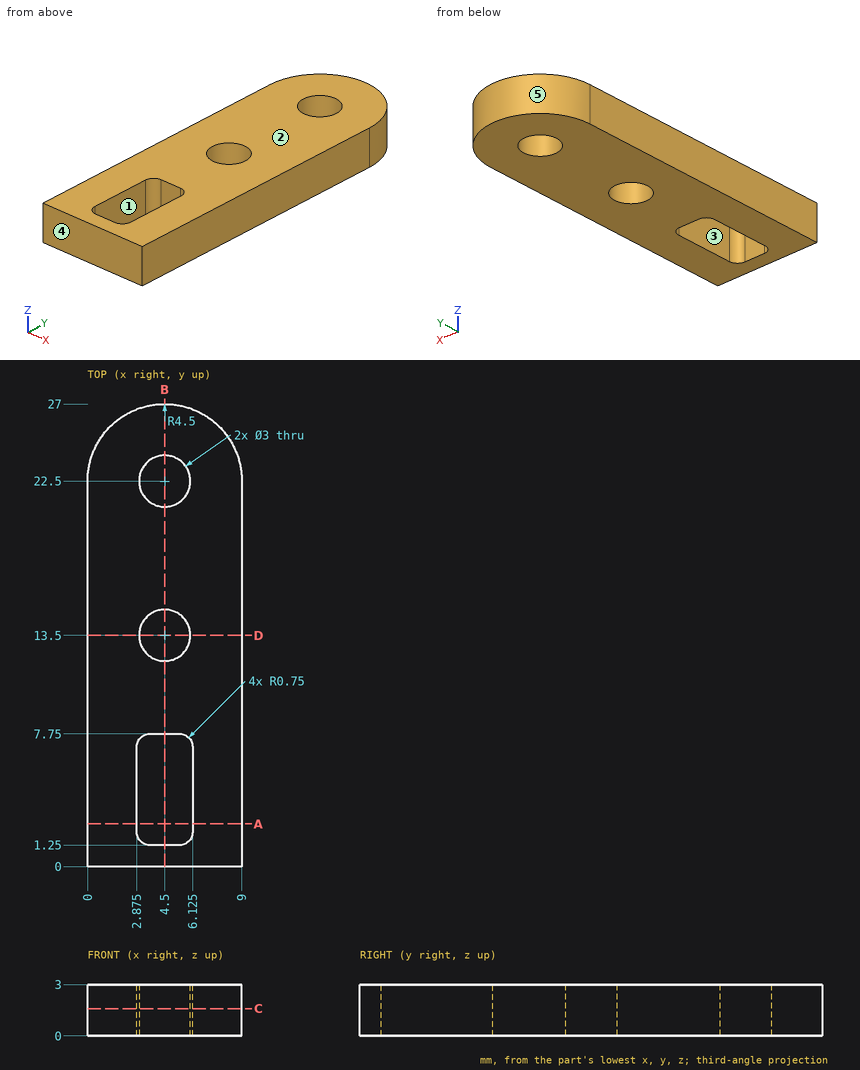
Here's the drawing with two shaded views (mm, measured from the low corner). I have some questions. A direction names the side the tool comes from. Coordinates: 2 decimals unless noted, no trailing zeros. Write each loop counter-clockwise with the first axis right and the second up, starting at its lowest first coordinate (ties: lowest second). Pieces come first, ordered by that corner, then holes. Notation, with made-up numbers: M 8,-25 L 63,-25 A30 ccw 63,12 Z; hole C -25.5,-27.75 d10. An arc over 180 degrees is marked long. Write item = value, one per line. Start each with the question number.
Q1. I'm going to push a flat-ended pin straight in: pin 1 (0.5 mm diameter, centred on x = 5, z = 1.5, fed in from +Y). Where does the tip first touch, or does it pass through?
Q2. If we section it at C-C, the plane z = 1.6: Write out the boundary of the cut face in (x, y) (3 decimals).
Q3. If we section it at D-D, the plane y = 13.5: Write out the boundary of the cut face in (x, z), then the cut area to 3 significant figures.
Q4. On a 3-axis mill with a long thin cutter (end or side, diameter ignored), from which of +Z, -Z, +X, -X, +Y, -Y can I reach the whole of each face in a straight line? I mean the marked faces 1 and 2. Say none if no direction works.
Q5. If we section it at B-B, the plane x = 4.5: Write out the boundary of the cut face in (y, z), then the cut area to 3 significant figures.
Q6. If we section it at A-A, the plane y = 2.5: Write out the boundary of the cut face in (x, z) (3 decimals).
Q7. If I drill on L1, parallel to Y at x = 4.5, z = 1.05; L2, parallel to Y at x = 3.5, z = 2.8; L3, parallel to X at y = 22.5, z = 0.8, over which ranges is the centre line in solid material (lowest first)? Write a range as [from, to].
Q8. Thinking about a two-plate mould opening in X: for the marked faces 3, 4 and 5, which applies, released by +X, released by -X, zero draft, split by the parting line, or undercut?
Check sheet entries:
q1.pin_1 = 26.99
q2.outline = M 0,0 L 9,0 L 9,22.5 A4.5 ccw 0,22.5 Z; hole M 2.875,2 A0.75 ccw 3.625,1.25 L 5.375,1.25 A0.75 ccw 6.125,2 L 6.125,7 A0.75 ccw 5.375,7.75 L 3.625,7.75 A0.75 ccw 2.875,7 Z; hole C 4.5,13.5 d3; hole C 4.5,22.5 d3
q3.outline = M 0,0 L 3,0 L 3,3 L 0,3 Z; M 6,0 L 9,0 L 9,3 L 6,3 Z
q3.area = 18.0 mm²
q4.face_1 = +Z, -Z
q4.face_2 = +Z, +X, -X, +Y, -Y
q5.outline = M 0,0 L 1.25,0 L 1.25,3 L 0,3 Z; M 7.75,0 L 12,0 L 12,3 L 7.75,3 Z; M 15,0 L 21,0 L 21,3 L 15,3 Z; M 24,0 L 27,0 L 27,3 L 24,3 Z
q5.area = 43.5 mm²
q6.outline = M 0,0 L 2.875,0 L 2.875,3 L 0,3 Z; M 6.125,0 L 9,0 L 9,3 L 6.125,3 Z
q7.L1 = [0, 1.25], [7.75, 12], [15, 21], [24, 27]
q7.L2 = [0, 1.26], [7.74, 12.38], [14.62, 21.38], [23.62, 26.89]
q7.L3 = [0, 3], [6, 9]
q8.face_3 = undercut
q8.face_4 = zero draft
q8.face_5 = split by the parting line
